Print and shaded views of the part. All mm, measured from the part's lowest x, y and z. A direction names the side the tool comes from. Round coordinates to 2 decimals unless told otherwise and drop trailing zeros. Loops run counter-clockwise (first coordinate to the right, second up) from the corner with the lowest first, then second, coordinate; pieces in that order, holes last. Notation, with made-up numbers: (85, 45) - (94, 45) arc R18 ccw to (94, 66) - close; hole circle Ø6 at (-2.5, 35.25). An arc over 180 degrees is marked (long way). Answer as a JSON object with one key per item and string values.
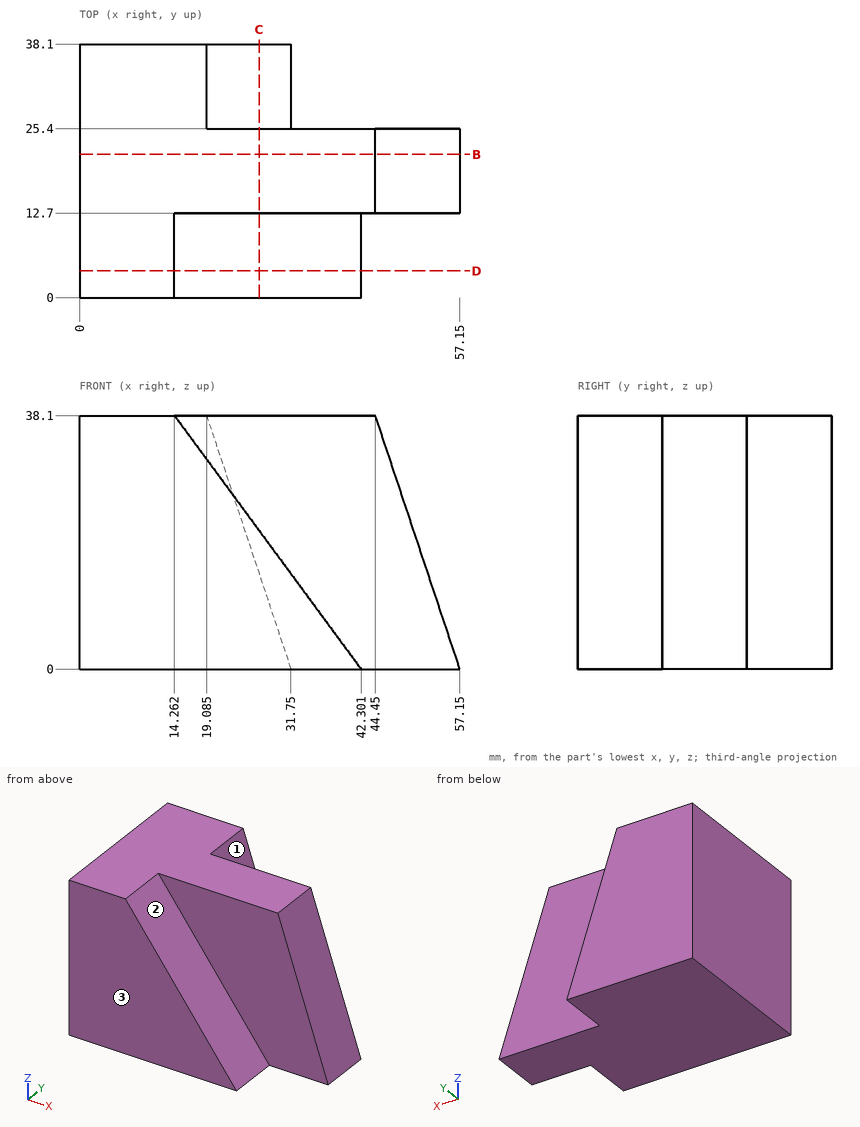
1) Drop flat-ended pins along their axis: P1, Ø6, axis at x = 18, z = 10, coming from the -Y side; P2, Ø3, axis at x = 48.5, z = 10.5, coming from the +Y side; P3, Ø10, axis at x = 35, z = 22.5, coming from the -Y side; P4, Ø6, axis at y = 29.5, z = 7.5, coming from the +X side. Give the stop position or say it passes through.
Values follow:
{"P1": "y = 0", "P2": "y = 25.4", "P3": "y = 12.7", "P4": "x = 30.25"}
2) Slice it at B-B on y = 21.5. List the corners of the cut face in (x, z).
Values follow:
{"outline": "(0, 0) - (57.15, 0) - (44.45, 38.1) - (0, 38.1) - close"}
3) Slice it at C-C on x = 27. List the corners of the cut face in (y, z).
Values follow:
{"outline": "(0, 0) - (38.1, 0) - (38.1, 14.29) - (25.4, 14.29) - (25.4, 38.1) - (12.7, 38.1) - (12.7, 20.79) - (0, 20.79) - close"}
4) Slice it at D-D on y = 4. List the corners of the cut face in (x, z), then the cut area to 3 significant figures.
Values follow:
{"outline": "(0, 0) - (42.3, 0) - (14.26, 38.1) - (0, 38.1) - close", "area": "1,080 mm²"}
5) Tool access for the marked faces 1, 2 and 3: list every direction of +Z, -Z, +X, -X, +Y, -Y with a clear straight run to the whole face (end or side of a thin tool).
Values follow:
{"face 1": "+Z, +X, +Y", "face 2": "+Z, +X, -Y", "face 3": "+Z, -Z, +X, -X, -Y"}
6) Probe probe 1 along Y at (x, z) = (47, 19); probe 2 along X at (y, z) = (12, 35) (1 decimal); probe 3 along X at (y, z) = (5, 35.5) (1 decimal). List the from-to ranges inside material, lowest first.
Values follow:
{"probe 1": "12.7 to 25.4", "probe 2": "0 to 16.5", "probe 3": "0 to 16.2"}
